The drawing under review shows one solid part. Ordinate dimensions are in mm from its lowest x, y, z. Coordinates: 2 decimals unless noted, no trailing zeros. Write each loop counter-clockwise with the first axis right and the second up, starting at its lowest first coordinate (ties: lowest second). Pieces come first, ordered by that corner, then holes.
Q1. Take a section at A-A (y = 2). Give the boundary of the cut face in (x, z).
Q2. Take a section at B-B (z = 24.5). Give the boundary of the cut face in (x, y), and give its area (3 significant figures).
Q3. Take a section at D-D (z = 11). Give the boundary of the cut face in (x, y).
Q4. For probe 1 along X at (y, z) = (3.3, 17.5); probe 2 along Z at (x, y) = (67.5, 2.2); probe 3 along X at (y, z) = (0.75, 26), list the stretches that pass through material, from the lowest coordinate up.
Q5. Take a section at C-C (x = 117). Give the boundary of the cut face in (y, z), and give its area (3 significant figures).
Q6. Insertion check: pin 1 (1.5 mm diameter, centred on x = 156.5, y = 2.5, fed in from +Z). The pin has a flat end and moves straight along its axis. Give the tip position at first contact, or say it passes through.
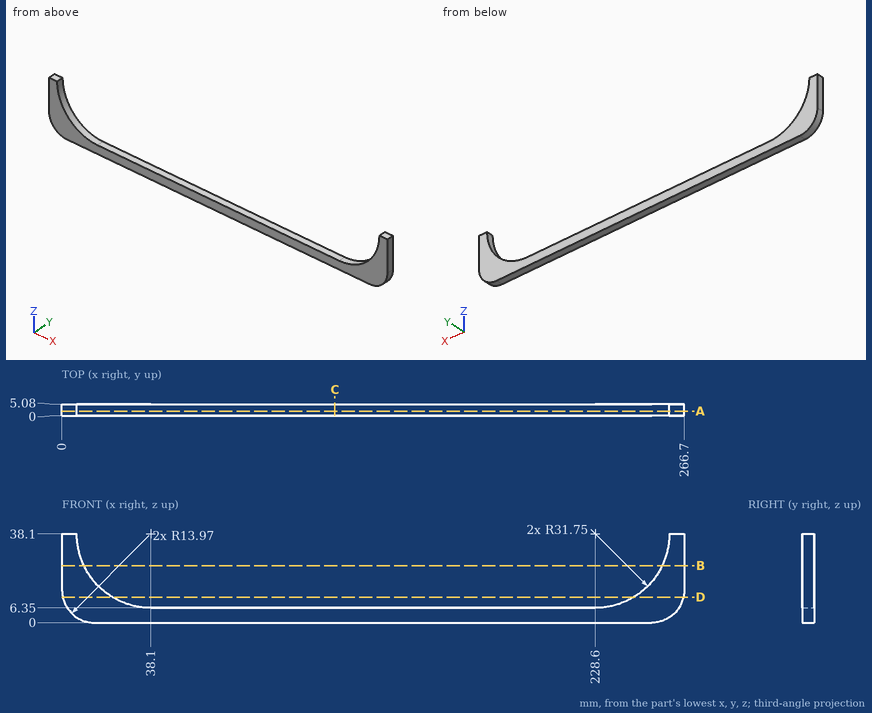
Response:
1. outline: (0, 13.97) arc R13.97 ccw to (13.97, 0) - (252.73, 0) arc R13.97 ccw to (266.7, 13.97) - (266.7, 38.1) - (260.35, 38.1) arc R31.75 cw to (228.6, 6.35) - (38.1, 6.35) arc R31.75 cw to (6.35, 38.1) - (0, 38.1) - close
2. outline: (0, 0) - (9.41, 0) - (9.41, 5.08) - (0, 5.08) - close; (257.29, 0) - (266.7, 0) - (266.7, 5.08) - (257.29, 5.08) - close
2. area: 95.6 mm2
3. outline: (0.32, 0) - (21.56, 0) - (21.56, 5.08) - (0.32, 5.08) - close; (245.14, 0) - (266.38, 0) - (266.38, 5.08) - (245.14, 5.08) - close
4. probe 1: x = 0 to 13.94, 252.76 to 266.7
4. probe 2: z = 0 to 6.35
4. probe 3: x = 0 to 8.75, 257.95 to 266.7
5. outline: (0, 0) - (5.08, 0) - (5.08, 6.35) - (0, 6.35) - close
5. area: 32.3 mm2
6. pin 1: stops at z = 6.35
